```python
from build123d import *

# Parameters (mm, degrees)
BOSS_EXTRUDE1_DEPTH = 4


with BuildPart() as part:
    # Sketch1 → Boss-Extrude1 (new body)
    with BuildSketch(Plane(origin=(0, -95.648578892, 0), x_dir=(-1, 0, 0), z_dir=(0, -1, 0))):
        with BuildLine():
            Line((-123.018568843, 257.712687792), (-116.306871964, 261.587687792))
            Line((-116.306871964, 261.587687792), (-86.056888913, 209.19318022))
            Line((-86.056888913, 209.19318022), (-82.592787298, 211.19318022))
            add(Edge.make_bspline(
                [(-82.592787298, 211.19318022), (-20.425563037, 110.136816529), (35.572246121, 110.775338662)],
                knots=[0, 0, 0, 1, 1, 1], degree=2))
            add(Edge.make_bspline(
                [(153.737279537, 211.193180221), (91.570055279, 110.136816529), (35.572246121, 110.775338662)],
                knots=[0, 0, 0, 1, 1, 1], degree=2))
            Line((153.737279537, 211.193180221), (157.201381153, 209.193180221))
            Line((157.201381153, 209.193180221), (187.451364204, 261.587687793))
            Line((187.451364204, 261.587687793), (194.163061083, 257.712687793))
            Line((194.163061083, 257.712687793), (163.913078032, 205.318180221))
            Line((163.913078032, 205.318180221), (167.377179647, 203.318180221))
            add(Edge.make_bspline(
                [(167.377179647, 203.318180221), (110.943413608, 98.951602883), (139.495294576, 50.775338663)],
                knots=[0, 0, 0, 1, 1, 1], degree=2))
            add(Edge.make_bspline(
                [(285.542213066, -1.349661336), (166.941222766, 1.960552309), (139.495294576, 50.775338663)],
                knots=[0, 0, 0, 1, 1, 1], degree=2))
            Line((285.542213066, -1.349661336), (285.542213066, -5.349661336))
            Line((285.542213066, -5.349661336), (346.042179168, -5.349661336))
            Line((346.042179168, -5.349661336), (346.042179168, -13.099661336))
            Line((346.042179168, -13.099661336), (285.542213066, -13.099661336))
            Line((285.542213066, -13.099661336), (285.542213066, -17.099661336))
            add(Edge.make_bspline(
                [(285.542213066, -17.099661336), (166.941222766, -20.409874983), (139.495294576, -69.224661337)],
                knots=[0, 0, 0, 1, 1, 1], degree=2))
            add(Edge.make_bspline(
                [(167.377179649, -221.767502894), (110.943413609, -117.400925558), (139.495294576, -69.224661337)],
                knots=[0, 0, 0, 1, 1, 1], degree=2))
            Line((167.377179649, -221.767502894), (163.913078034, -223.767502894))
            Line((163.913078034, -223.767502894), (194.163061085, -276.162010466))
            Line((194.163061085, -276.162010466), (187.451364206, -280.037010466))
            Line((187.451364206, -280.037010466), (157.201381155, -227.642502894))
            Line((157.201381155, -227.642502894), (153.737279539, -229.642502894))
            add(Edge.make_bspline(
                [(153.737279539, -229.642502894), (91.57005528, -128.586139204), (35.572246122, -129.224661338)],
                knots=[0, 0, 0, 1, 1, 1], degree=2))
            add(Edge.make_bspline(
                [(-82.592787296, -229.642502896), (-20.425563036, -128.586139204), (35.572246122, -129.224661338)],
                knots=[0, 0, 0, 1, 1, 1], degree=2))
            Line((-82.592787296, -229.642502896), (-86.056888911, -227.642502895))
            Line((-86.056888911, -227.642502895), (-116.306871962, -280.037010467))
            Line((-116.306871962, -280.037010467), (-123.018568841, -276.162010467))
            Line((-123.018568841, -276.162010467), (-92.76858579, -223.767502895))
            Line((-92.76858579, -223.767502895), (-96.232687406, -221.767502895))
            add(Edge.make_bspline(
                [(-96.232687406, -221.767502895), (-39.798921364, -117.400925558), (-68.350802332, -69.224661338)],
                knots=[0, 0, 0, 1, 1, 1], degree=2))
            add(Edge.make_bspline(
                [(-214.397720824, -17.099661339), (-95.796730523, -20.409874984), (-68.350802332, -69.224661338)],
                knots=[0, 0, 0, 1, 1, 1], degree=2))
            Line((-214.397720824, -17.099661339), (-214.397720824, -13.099661338))
            Line((-214.397720824, -13.099661338), (-274.897686926, -13.099661338))
            Line((-274.897686926, -13.099661338), (-274.897686926, -5.349661338))
            Line((-274.897686926, -5.349661338), (-214.397720824, -5.349661338))
            Line((-214.397720824, -5.349661338), (-214.397720824, -1.349661338))
            add(Edge.make_bspline(
                [(-214.397720824, -1.349661338), (-95.796730523, 1.960552308), (-68.350802333, 50.775338662)],
                knots=[0, 0, 0, 1, 1, 1], degree=2))
            add(Edge.make_bspline(
                [(-96.232687408, 203.31818022), (-39.798921365, 98.951602882), (-68.350802333, 50.775338662)],
                knots=[0, 0, 0, 1, 1, 1], degree=2))
            Line((-96.232687408, 203.31818022), (-92.768585792, 205.31818022))
            Line((-92.768585792, 205.31818022), (-123.018568843, 257.712687792))
        make_face()
        Polygon((9.149169363, -55.090772776), (-3.656970853, -77.271658278), (-0.192869237, -79.271658278), (-2.192869237, -82.735759893), (-5.656970853, -80.735759893), (-11.656970853, -91.128064739), (-15.207675008, -89.078064739), (-9.207675008, -78.685759893), (-12.671776623, -76.685759893), (-10.671776623, -73.221658278), (-7.207675008, -75.221658278), (5.598465207, -53.040772776), align=None, mode=Mode.SUBTRACT)
    extrude(amount=BOSS_EXTRUDE1_DEPTH)


solid = part.part
```
Source: CAD feature listing. Evaluate the final solid. Frame: model axes, mm. A direction names the side the tool comes from. Round coordinates to 2 decimals unless told otherwise and drop trailing zeros. Loops run counter-clockwise (first coordinate to the right, second up) from the corner with the lowest first, then second, coordinate; pieces in that order, holes last.
1. Mould query, pull axis X, two halves, no side actions, for faces 5 (the flat face through (107.682, -97.621, -231.149)), 6 (the flat face through (-37, -95.649, 8)), 7 (the flat face through (0.9, -97.6, 64.3)). Classes: released by +X, released by -X, zero draft, split by the parting line, or undercut.
2. Access query for faces 1 (the flat face through (-172.54, -97.62, 254.21)), 2 (the flat face through (108.105, -97.621, 250.332)), 3 (the flat face through (-179.25, -97.62, -231.88)), 4 (the flat face through (101.394, -97.621, -235.757)). Directions: +Z, -Z, +X, -X, +Y, -Y. A direction counts if a zero-diameter tool reaches every point of the face in a straight line with its end or side. Return the directions, or none.
3. Section query A-A on z = -219. Output: boundary loops of the cut face in (x, y).
4. Ray query, L1, parallel to Z at x = 79, y = -98.65; L2, parallel to Z at x = 112, y = -99.05; L3, parallel to X at y = -98.7, z = -142. Return the intervals inside material, ascending.
5. Contact query for flat-ended pins moving along their axis: pin 1 (2 mm diameter, centred on x = 236, y = -98, fed in from +Z); pin 2 (2 mm diameter, centred on y = -97.5, z = 14.5, fed in from -X); pin 3 (1.5 mm diameter, centred on y = -99, z = -131, fed in from -X). Output: stop coordinate, or through.
6. Section query B-B on x = -178. Give the number of separate pieces and of enclosed holes in the cut face, and give its area (3 significant figures).
Answers below:
1. face 5: released by +X
1. face 6: zero draft
1. face 7: undercut
2. face 1: +Z, +Y, -Y
2. face 2: +X, +Y, -Y
2. face 3: -X, +Y, -Y
2. face 4: -Z, +Y, -Y
3. outline: (-171.81, -99.65) - (-162.86, -99.65) - (-162.86, -95.65) - (-171.81, -95.65) - close; (91.72, -99.65) - (100.67, -99.65) - (100.67, -95.65) - (91.72, -95.65) - close
4. L1: z = -205.43 to -168.32, -36.79 to 55.23, 186.77 to 223.88
4. L2: z = -254.13 to -238.63, -15.86 to 34.3, 257.08 to 272.58
4. L3: x = -139.87 to -100.28, 29.13 to 68.72
5. pin 1: stops at z = 13.1
5. pin 2: stops at x = -285.54
5. pin 3: stops at x = -136.65
6. separate pieces: 3
6. enclosed holes: 0
6. area: 342 mm2
